Can you work these out from the model? Positions are in its coordinate system, mm. Face numbers are marked on the shaded views. A direction names the side the tool comes from. Give positions to 0.01 mm unless a question says otherwise; leave off trailing zeros. Loops run counter-clockwise (first coordinate to the right, second up) from the corner with the lowest first, then second, coordinate; pieces in that order, holes last. Notation, with made-up numbers: (61, 44) - (66, 44) arc R34 ccw to (66, 79) - close; hole circle Ø8 at (27.5, 72). An arc over 180 degrees is marked (long way). Use a Markdown table: item, result. Add a question column.
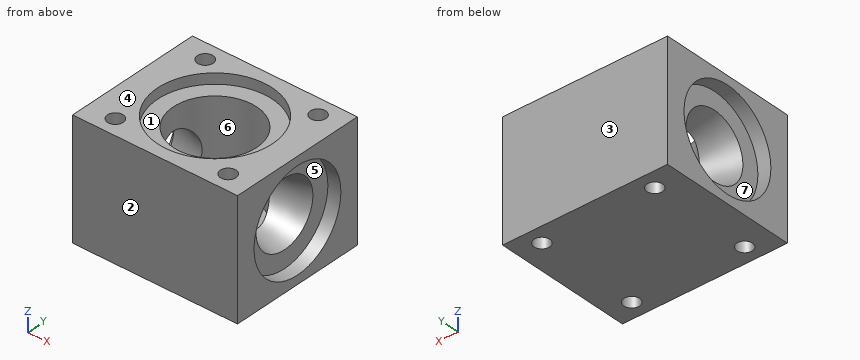
```python
from build123d import *

# Parameters (mm, degrees)
F0_W     = 95
F0_H     = 80
F1_DEPTH = 34
F4_R     = 4.5
F5_DEPTH = 68
F4_R_2   = 24
F6_DEPTH = 57
F4_R_3   = 33
F7_DEPTH = 6


with BuildPart() as f1:
    # F0 (on Top) → F1 (new body, symmetric)
    with BuildSketch(Plane.XY):
        Rectangle(F0_W, F0_H)
    extrude(amount=F1_DEPTH, both=True)

    # F2 (on Front) → F3 (revolve, cut)
    with BuildSketch(Plane.XZ):
        Polygon((47.5, 0), (47.5, 29), (40, 29), (40, 19), (10, 11.730042), (-10, 11.730042), (-40, 19), (-40, 29), (-47.5, 29), (-47.5, 0), align=None)
    revolve(axis=Axis((-0.459014, 0, 0), (1, 0, 0)), mode=Mode.SUBTRACT)

    # F4 (on face) → F5 (cut)
    with BuildSketch(Plane.XY.offset(34)):
        with Locations((-31.5, 30)):
            Circle(F4_R)
        with Locations((33.5, 30)):
            Circle(F4_R)
        with Locations((-31.5, -30)):
            Circle(F4_R)
        with Locations((33.5, -30)):
            Circle(F4_R)
    extrude(amount=-F5_DEPTH, mode=Mode.SUBTRACT)

    # F4 (on face) → F6 (cut)
    with BuildSketch(Plane.XY.offset(34)):
        Circle(F4_R_2)
    extrude(amount=-F6_DEPTH, mode=Mode.SUBTRACT)

    # F4 (on face) → F7 (cut)
    with BuildSketch(Plane.XY.offset(34)):
        Circle(F4_R_3)
        Circle(F4_R_2, mode=Mode.SUBTRACT)
    extrude(amount=-F7_DEPTH, mode=Mode.SUBTRACT)


solid = f1.part
```
1. If we mould it in two halves opening along Y, with no side actions, what happens to the marked faces 1, 2 and 3? For each: released by +Y, released by -Y, zero draft, split by the parting line, or undercut.
2. Suppose I cut it at D-D (z = -13). State how many separate pieces and enclosed holes the cut face has, and give its area (3 significant figures).
3. On a 3-axis mill with a long thin cutter (end or side, diameter ignored), from which of +Z, -Z, +X, -X, +Y, -Y can I reach the whole of each face in a straight line? I mean the marked faces 4, 5, 6 and 7. Say none if no direction works.
4. Suppose I cut it at B-B (y = 0). List the corners of the cut face in (x, z) for me, and give its area (3 significant figures).
5. Suppose I cut it at A-A (x = 30.5). List the corners of the cut face in (y, z) for me, and give its area (3 significant figures).
6. Will these pins go through, and if not, where does the flat tip stop? P1, Ø1, axis at x = 32, y = -28, coming from the +Z side; P2, Ø24, axis at x = -10.5, y = 0.5, coming from the +Z side; P3, Ø17.5, axis at y = -13, z = 8.5, coming from the -X side.
7. Suppose I cut it at C-C (x = 0). List the corners of the cut face in (y, z) for me, and give its area (3 significant figures).
8. Please list where these lines run through material, in increasing order: line 1 along X through (y, z) = (14, -20); line 2 along Z through (x, y) = (41, 1); line 3 along Y through (x, z) = (-34, -9.5). Write a range as [from, to].
Results below:
| question | item | result |
|---|---|---|
| 1 | face 1 | undercut |
| 1 | face 2 | released by -Y |
| 1 | face 3 | released by +Y |
| 2 | separate pieces | 2 |
| 2 | enclosed holes | 4 |
| 2 | area | 4,040 mm² |
| 3 | face 4 | +Z, +X, -X, +Y, -Y |
| 3 | face 5 | +X |
| 3 | face 6 | +Z |
| 3 | face 7 | -X |
| 4 | outline | (-47.5, -34) - (47.5, -34) - (47.5, -29) - (40, -29) - (40, -19) - (24, -15.12) - (24, -23) - (-24, -23) - (-24, -15.12) - (-40, -19) - (-40, -29) - (-47.5, -29) - close; (-47.5, 29) - (-40, 29) - (-40, 19) - (-24, 15.12) - (-24, 28) - (-33, 28) - (-33, 34) - (-47.5, 34) - close; (24, 15.12) - (40, 19) - (40, 29) - (47.5, 29) - (47.5, 34) - (33, 34) - (33, 28) - (24, 28) - close |
| 4 | area | 1,650 mm² |
| 5 | outline | (-40, -34) - (-33.35, -34) - (-33.35, 34) - (-40, 34) - close; (-26.65, -34) - (26.65, -34) - (26.65, 34) - (12.6, 34) - (12.6, 28) - (-12.6, 28) - (-12.6, 34) - (-26.65, 34) - close; (33.35, -34) - (40, -34) - (40, 34) - (33.35, 34) - close; hole circle Ø33.4 at (0, 0) |
| 5 | area | 3,500 mm² |
| 6 | P1 | through |
| 6 | P2 | z = -23 |
| 6 | P3 | x = -40 |
| 7 | outline | (-40, -34) - (40, -34) - (40, 34) - (33, 34) - (33, 28) - (24, 28) - (24, -23) - (-24, -23) - (-24, 28) - (-33, 28) - (-33, 34) - (-40, 34) - close |
| 7 | area | 2,600 mm² |
| 8 | line 1 | [-40, -19.49], [19.49, 40] |
| 8 | line 2 | [-34, -28.98], [28.98, 34] |
| 8 | line 3 | [-40, -33.74], [-26.26, -14.75], [14.75, 26.26], [33.74, 40] |
